```python
from build123d import *

# Parameters (mm, degrees)
ESBO_O1_W                = 65
ESBO_O1_H                = 40
RESSALTO_EXTRUS_O1_DEPTH = 30
ESBO_O2_W                = 61
ESBO_O2_H                = 37
CORTE_EXTRUS_O1_DEPTH    = 20
ESBO_O3_W                = 61
ESBO_O3_H                = 27
CORTE_EXTRUS_O2_DEPTH    = 49
ESBO_O5_W                = 61
ESBO_O5_H                = 1.5
CORTE_EXTRUS_O3_DEPTH    = 49
ESBO_O7_R                = 5
RESSALTO_EXTRUS_O2_DEPTH = 4
ESBO_O8_R                = 1.6
RESSALTO_EXTRUS_O3_DEPTH = 6
ESBO_O10_R               = 3.5
RESSALTO_EXTRUS_O4_DEPTH = 6
ESBO_O12_R               = 2.75
CORTE_EXTRUS_O4_DEPTH    = 4


with BuildPart() as part:
    # Esboço1 → Ressalto-extrusão1 (new body)
    with BuildSketch(Plane.XY):
        Rectangle(ESBO_O1_W, ESBO_O1_H)
    extrude(amount=RESSALTO_EXTRUS_O1_DEPTH)

    # Esboço2 → Corte-extrusão1 (cut)
    with BuildSketch(Plane(origin=(0, 0, 0), x_dir=(-1, 0, 0), z_dir=(0, 0, -1))):
        Rectangle(ESBO_O2_W, ESBO_O2_H)
    extrude(amount=-CORTE_EXTRUS_O1_DEPTH, mode=Mode.SUBTRACT)

    # Esboço3 → Corte-extrusão2 (cut)
    with BuildSketch(Plane(origin=(0, 20, 0), x_dir=(1, 0, 0), z_dir=(0, 1, 0))):
        with Locations((0, -15)):
            Rectangle(ESBO_O3_W, ESBO_O3_H)
    extrude(amount=-CORTE_EXTRUS_O2_DEPTH, mode=Mode.SUBTRACT)

    # Esboço5 → Corte-extrusão3 (cut)
    with BuildSketch(Plane(origin=(0, 20, 0), x_dir=(1, 0, 0), z_dir=(0, 1, 0))):
        with Locations((0, -0.75)):
            Rectangle(ESBO_O5_W, ESBO_O5_H)
    extrude(amount=-CORTE_EXTRUS_O3_DEPTH, mode=Mode.SUBTRACT)

    # Esboço7 → Ressalto-extrusão2 (add)
    with BuildSketch(Plane.ZY.offset(32.5)):
        with Locations((6.224890869, 0)):
            Circle(ESBO_O7_R)
    extrude(amount=-RESSALTO_EXTRUS_O2_DEPTH)

    # Esboço8 → Ressalto-extrusão3 (add)
    with BuildSketch(Plane(origin=(-28.5, 0, 0), x_dir=(0, 0, -1), z_dir=(1, 0, 0))):
        with Locations((-6.224890869, 0)):
            Circle(ESBO_O8_R)
    extrude(amount=RESSALTO_EXTRUS_O3_DEPTH)

    # Esboço10 → Ressalto-extrusão4 (add)
    with BuildSketch(Plane(origin=(32.5, 0, 0), x_dir=(0, 0, -1), z_dir=(1, 0, 0))):
        with Locations(Location((-6.224890869, 0, 0), (0, 0, 90))):
            Circle(ESBO_O10_R)
    extrude(amount=-RESSALTO_EXTRUS_O4_DEPTH)

    # Esboço12 → Corte-extrusão4 (cut)
    with BuildSketch(Plane.ZY.offset(-26.5)):
        with Locations(Location((6.224890869, 0, 0), (0, 0, 270))):
            Circle(ESBO_O12_R)
    extrude(amount=-CORTE_EXTRUS_O4_DEPTH, mode=Mode.SUBTRACT)


solid = part.part
```
Geometry: final body of the model. Coordinates: model frame, mm. A direction names the side the tool comes from. Round coordinates to 2 decimals unless told otherwise and drop trailing zeros. Order: outer loops, then holes, each group sorted by start corner. A loop starts at its lowest first (then second) coordinate and runs counter-clockwise, first axis right, second up. Notation, with made-up numbers: (9, 20) -> (19, 20) arc R10 cw to (19, 32) -> close; hole circle Ø7 at (58, 20.5). An arc over 180 degrees is marked (long way). Use CSV: the item, a comma, the result in double quotes. Start each with the question number.
1) First-contact query: pin 1 Ø8 at (x, z) = (7.5, 26) entering from +Y; pin 2 Ø5 at (x, y) = (-26, 9.5) entering from -Z. Flat tips, straight axial feed; report the tip coordinate or a pass-through.
2) Material intervals for line 1 along Z through (x, y) = (27, 0); line 2 along X through (y, z) = (-14.5, 23.75); line 3 along X through (y, z) = (1, 8.5), sorted ascending. Write a range as from..to.
3) Section C-C (z = 5.5). Return the cut outline in (x, y), and give its area (3 significant figures).
4) Set-up query: faces 5 (the face through (0, -20, 29)), 6 (the face through (-29.514, 1.502, 10.994)). Return all of +Z, -Z, +X, -X, +Y, -Y with unobstructed straight access to the full face (end or side cutting, diameter ignored); none if empty.
5) Section D-D (y = 0). Return the cut outline in (x, z), and give its area (3 significant figures).
6) Section B-B (y = 9). Return the cut outline in (x, z).
7) Draft query along X for faces 1 (the face through (0, 0, 30)), 2 (the face through (-22.5, 0, 6)), 3 (the face through (32.5, 0, 15)), 4 (the face through (26.5, -2, 4)). Return one class per face: +X half, -X half, draft (parallel to the pull), parting line (faces both ways), or undercut.
8) Section A-A (z = 16.25). Return the cut outline in (x, y).
Returned:
1,pin 1,"stops at y = 20"
1,pin 2,"stops at z = 28.5"
2,line 1,"z = 2.72..3.47, 8.97..9.72, 28.5..30"
2,line 2,"x = -32.5..-30.5, 30.5..32.5"
2,line 3,"x = -32.5..-28.5, 30.5..32.5"
3,outline,"(-32.5, -20) -> (-30.5, -20) -> (-30.5, -4.95) -> (-28.5, -4.95) -> (-28.5, -1.43) -> (-22.5, -1.43) -> (-22.5, 1.43) -> (-28.5, 1.43) -> (-28.5, 4.95) -> (-30.5, 4.95) -> (-30.5, 20) -> (-32.5, 20) -> close; (26.5, -3.42) -> (30.5, -3.42) -> (30.5, -20) -> (32.5, -20) -> (32.5, 20) -> (30.5, 20) -> (30.5, 3.42) -> (26.5, 3.42) -> (26.5, 2.65) -> (30.5, 2.65) -> (30.5, -2.65) -> (26.5, -2.65) -> close"
3,area,"203 mm²"
4,face 5,"+Z, -Z, +X, -X, -Y"
4,face 6,"none"
5,outline,"(-32.5, 0) -> (-30.5, 0) -> (-30.5, 1.22) -> (-28.5, 1.22) -> (-28.5, 4.62) -> (-22.5, 4.62) -> (-22.5, 7.82) -> (-28.5, 7.82) -> (-28.5, 11.22) -> (-30.5, 11.22) -> (-30.5, 28.5) -> (30.5, 28.5) -> (30.5, 9.72) -> (26.5, 9.72) -> (26.5, 8.97) -> (30.5, 8.97) -> (30.5, 3.47) -> (26.5, 3.47) -> (26.5, 2.72) -> (30.5, 2.72) -> (30.5, 0) -> (32.5, 0) -> (32.5, 30) -> (-32.5, 30) -> close"
5,area,"257 mm²"
6,outline,"(-32.5, 0) -> (-30.5, 0) -> (-30.5, 28.5) -> (30.5, 28.5) -> (30.5, 0) -> (32.5, 0) -> (32.5, 30) -> (-32.5, 30) -> close"
7,face 1,"draft"
7,face 2,"undercut"
7,face 3,"+X half"
7,face 4,"undercut"
8,outline,"(-32.5, -20) -> (-30.5, -20) -> (-30.5, 20) -> (-32.5, 20) -> close; (30.5, -20) -> (32.5, -20) -> (32.5, 20) -> (30.5, 20) -> close"
